Autodesk Inventor part; units mm, degrees
ref_plane "YZ Plane" through (0, 0, 0) normal (1, 0, 0) x (0, 1, 0)
ref_plane "XZ Plane" through (0, 0, 0) normal (0, 1, 0) x (-1, 0, 0)
ref_plane "XY Plane" through (0, 0, 0) normal (0, 0, 1) x (1, 0, 0)
sketch "Sketch1" plane through (0, 0, 0) normal (1, 0, 0) x (0, 1, 0)
  circle A0 centre (0, 0) radius 37.5
  dimension "d0" = 75
extrude "Extrusion1" add sketch "Sketch1" along normal mid plane 53
sketch "Sketch2" plane through (26.5, 0, 0) normal (1, 0, 0) x (0, 0, -1)
  circle A0 centre (0, 0) radius 14
  dimension "d3" = 28
extrude "Extrusion2" cut sketch "Sketch2" against normal blind 17.5
ref_plane "Work Plane1" through (16, 0, 0) normal (1, 0, 0) x (0, 0, -1)
sketch "Sketch3" plane through (0, 0, 0) normal (0, 0, 1) x (1, 0, 0)
  line L0 (-26.5, 37.5) -> (26.5, 37.5)
  line L1 (26.5, -37.5) -> (26.5, 37.5)
  line L2 (16, 52.5) -> (16, -52.5)
  line L3 (26.5, 33.5) -> (-26.5, 33.5)
  line L4 (-26.5, 37.5) -> (-26.5, -37.5)
  line L5 (26.5, 14) -> (9, 14)
  line L6 (16, 14) -> (26.5, 33.5)
  line L7 (-37.1, 0) -> (37.1, 0)
  point P0 (0, 0)
  dimension "d7" = 4
revolve "Revolution1" cut sketch "Sketch3" angle 360 about axis through (-10, 0, 0) along (1, 0, 0) contours L1 L5 L6
sketch "Sketch4" plane through (9, 0, 0) normal (1, 0, 0) x (0, 0, -1)
  circle A0 centre (0, 0) radius 11
  dimension "d9" = 22
extrude "Extrusion3" cut sketch "Sketch4" against normal through all
sketch "Sketch5" plane through (-26.5, 0, 0) normal (-1, 0, 0) x (0, 0, 1)
  circle A0 centre (0, 0) radius 28.5
  circle A1 centre (0, 0) radius 37.5
  dimension "d13" = 9
ref_plane "Work Plane2" through (-17, 0, 0) normal (1, 0, 0) x (0, 0, -1)
sketch "Sketch6" plane through (0, 0, 0) normal (0, 0, 1) x (1, 0, 0)
  line L0 (-26.5, 28.5) -> (-26.5, -28.5)
  line L1 (9, 11) -> (-26.5, 11)
  line L2 (-17, 52.5) -> (-17, -52.5)
  line L3 (-17, 11) -> (-26.5, 28.5)
  line L4 (-37.1, 0) -> (37.1, 0)
  point P0 (0, 0)
revolve "Revolution2" cut sketch "Sketch6" angle 360 about axis through (-10, 0, 0) along (1, 0, 0) contours L3 L1 L0
properties part number "LongboardWheel_RI" material "Nylon 6/6"
Can you work these out from the model? Positions are in its coordinate system, mm. A direction names the side the tool comes from. Give positions to 0.01 mm unless a question says otherwise; leave off trailing zeros. Order: outer loops, then holes, each group sorted by start corner. A loop starts at its lowest first (then second) coordinate and runs counter-clockwise, first axis right, second up. Notation, with made-up numbers: M 82.25,-27 L 86.25,-27 A21 cw 86.25,6 Z; hole C 55,25.25 d6. An arc over 180 degrees is marked long. One line per item, written item: value.
1) On a 3-axis mill with a long thin cutter (end or side, diameter ignored), from which of +Z, -Z, +X, -X, +Y, -Y can I reach the whole of each face in a straight line? I mean faces 1 (the face through (9, -9.3, -6.2)), 2 (the face through (-26.5, 25, 14)). Say none if no direction works.
Answer sheet:
face 1: +X
face 2: +Z, -Z, -X, +Y, -Y
2) Please list where these lines run through material, in increasing order: line 1 along Z through (x, y) = (-5, 0); line 2 along Z through (x, y) = (11, 0); line 3 along Y through (x, z) = (14, 11).
Answer sheet:
line 1: z = -37.5 to -11, 11 to 37.5
line 2: z = -37.5 to -14, 14 to 37.5
line 3: y = -35.85 to -8.66, 8.66 to 35.85
3) For P1, Ø1, axis at y = -17, z = -17.5, coming from the -X side; P2, Ø3, axis at x = -17.5, z = 17, coming from the -Y side; P3, Ø25, axis at y = 0, z = 0, coming from the +X side, each with a flat end and sliding along its axis, tell me the tip position at first contact or that it passes through.
Answer sheet:
P1: stops at x = -24.54
P2: stops at y = -34.15
P3: stops at x = 9
4) I want a section at A-A, the plane z = 0. List the corners of the cut face in (x, y) for me, plus the area to 3 significant figures.
Answer sheet:
outline: M -26.5,-37.5 L 26.5,-37.5 L 26.5,-33.5 L 16,-14 L 9,-14 L 9,-11 L -17,-11 L -26.5,-28.5 Z; M -26.5,28.5 L -17,11 L 9,11 L 9,14 L 16,14 L 26.5,33.5 L 26.5,37.5 L -26.5,37.5 Z
area: 2,330 mm^2
5) I want a section at C-C, the plane x = 19.5. List the corners of the cut face in (y, z) for me, plus the area to 3 significant figures.
Answer sheet:
outline: C 0,0 d75; hole C 0,0 d41
area: 3,100 mm^2
6) We'd pull the mould along Z, two halves only. Please class faces 3 (the face through (-3.82, -10.74, 2.38)), 4 (the face through (-0.37, -4.88, -37.18)), 5 (the face through (26.5, -14, 31)), 6 (the face through (16.66, -3.3, -14.86)): released by +Z, released by -Z, zero draft, split by the parting line, or undercut.
Answer sheet:
face 3: undercut
face 4: split by the parting line
face 5: zero draft
face 6: undercut
7) I want a section at D-D, the plane x = -2. List the corners of the cut face in (y, z) for me.
Answer sheet:
outline: C 0,0 d75; hole C 0,0 d22
